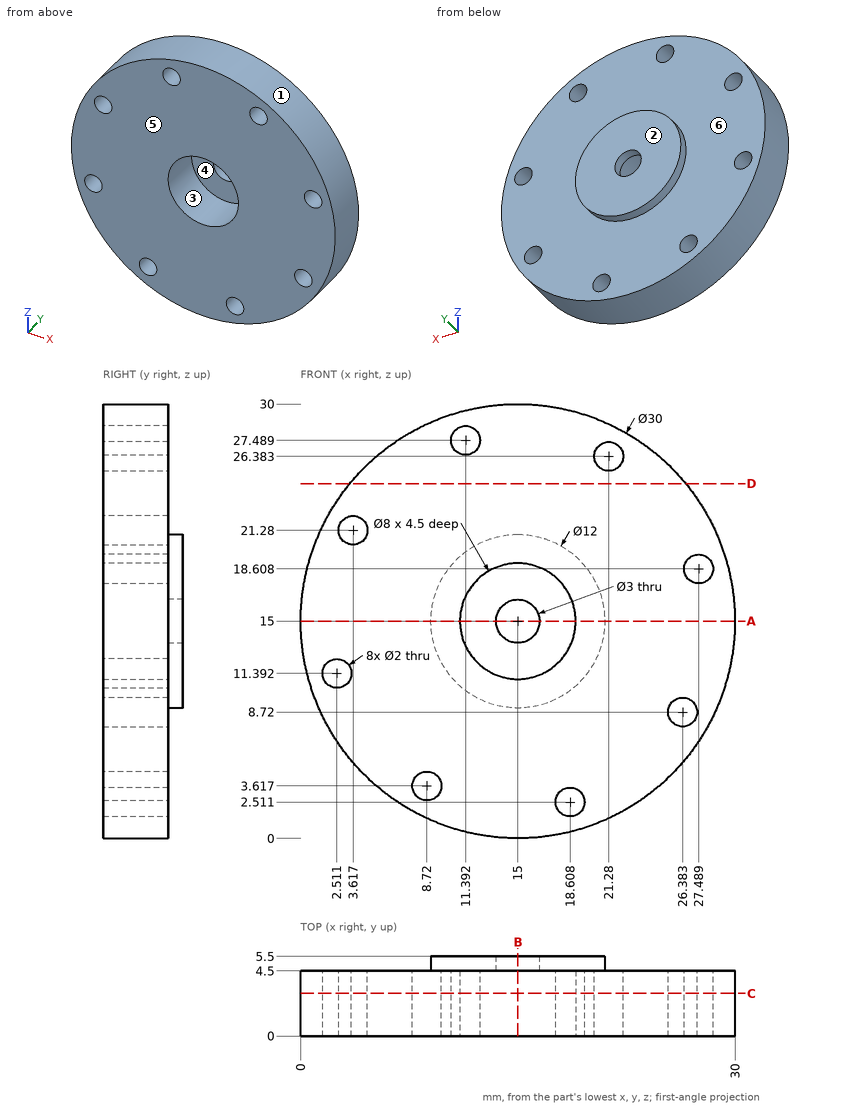
Design review of the part shown in the three views and the two pictorial views. Dimensions are in mm from the part's minimum x, y and z. A direction names the side the tool comes from. Round coordinates to 2 decimals unless told otherwise and drop trailing zeros. Write each loop counter-clockwise with the first axis right and the second up, starting at its lowest first coordinate (ties: lowest second). Pieces come first, ordered by that corner, then holes. Notation, with made-up numbers: (5, 87.25) -> (9, 87.25) arc R23 ccw to (9, 121.25) -> close; hole circle Ø1 at (20.5, 12). An arc over 180 degrees is marked (long way). Write item = value, one per line. Start each with the question number.
1) Take a section at D-D, the plane z = 24.5. State the section outline as (x, y) points.
2) Tool access review of the marked faces 4, 5 and 6: name each direction out of +Z, -Z, +X, -X, +Y, -Y from which nothing blocks a thin tool from reaching the whole face with its end or side.
3) Wall thickness on probe 1 along Z at (x, y) = (27, 4.1) (1 decimal); probe 2 along X at (y, z) = (3.5, 15); probe 3 along Y at (x, z) = (23, 21.5): over which ranges is each line inside the solid? List them lowest first. Write a range as from..to.
4) Clearance check with flat-ended pins moving along their axes: pin 1 (6.5 mm diameter, centred on x = 13.5, z = 13, fed in from -Y); pin 2 (6.5 mm diameter, centred on x = 15, z = 15, fed in from -Y); pin 3 (2.5 mm diameter, centred on x = 18.61, z = 2.51, fed in from +Y); pin 4 (1 mm diameter, centred on y = 4, z = 23.5, fed in from +X). State where each tip first meets the part, or that it passes through.
5) Take a section at A-A, the plane z = 15. State the section outline as (x, y) points.
6) Take a section at C-C, the plane y = 2.95. Count the separate pieces of the cut face and the enclosed holes in it.
7) Take a section at B-B, the plane x = 15. State the section outline as (y, z) points.
8) Mouldability with a two-part tool opening along Z and no side actions: class the marked faces 1, 2 and 3 as +Z half, -Z half, draft (parallel to the pull), parting line (faces both ways), or undercut.
Results list:
q1.outline = (3.39, 0) -> (26.61, 0) -> (26.61, 4.5) -> (3.39, 4.5) -> close
q2.face_4 = -Y
q2.face_5 = +Z, -Z, +X, -X, -Y
q2.face_6 = +Y
q3.probe_1 = 6..7.9, 9.5..17.7, 19.5..24
q3.probe_2 = 0..11, 19..30
q3.probe_3 = 0..4.5
q4.pin_1 = 0
q4.pin_2 = 4.5
q4.pin_3 = 4.5
q4.pin_4 = 27.69
q5.outline = (0, 0) -> (11, 0) -> (11, 4.5) -> (13.5, 4.5) -> (13.5, 5.5) -> (9, 5.5) -> (9, 4.5) -> (0, 4.5) -> close; (16.5, 4.5) -> (19, 4.5) -> (19, 0) -> (30, 0) -> (30, 4.5) -> (21, 4.5) -> (21, 5.5) -> (16.5, 5.5) -> close
q6.separate_pieces = 1
q6.enclosed_holes = 9
q7.outline = (0, 0) -> (4.5, 0) -> (4.5, 9) -> (5.5, 9) -> (5.5, 13.5) -> (4.5, 13.5) -> (4.5, 11) -> (0, 11) -> close; (0, 19) -> (4.5, 19) -> (4.5, 16.5) -> (5.5, 16.5) -> (5.5, 21) -> (4.5, 21) -> (4.5, 30) -> (0, 30) -> close
q8.face_1 = parting line
q8.face_2 = draft
q8.face_3 = undercut
